Geometry: final body of the model. Coordinates: model frame, mm. Face numbers are marked on the shaded views. A direction names the side the tool comes from. Round coordinates to 2 decimals unless told otherwise and drop trailing zeros. Write each loop counter-clockwise with the first axis right and the second up, starting at its lowest first coordinate (ties: lowest second). Pieces come first, ordered by that corner, then holes. Notation, with made-up numbers: (58, -17.5) - (79, -17.5) arc R31 ccw to (79, 15.5) - close; hole circle Ø6 at (17, 78.5). An arc over 180 degrees is marked (long way). Use a Markdown table: item, result. Add a question column.
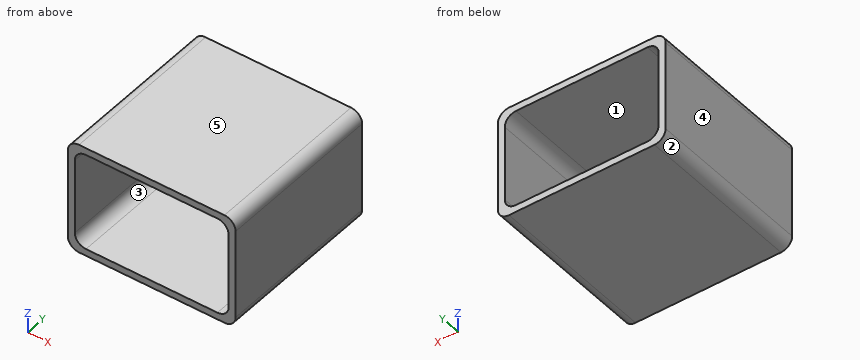
```python
from build123d import *

# Parameters (mm, degrees)
F0_W     = 76.2
F0_H     = 50.8
F1_DEPTH = 76.2
F2_T     = -3.175
F3_R     = 5.08


with BuildPart() as f1:
    # F0 (on Front) → F1 (new body)
    with BuildSketch(Plane.XZ):
        with Locations((7.1646266146, -4.8404615372)):
            Rectangle(F0_W, F0_H)
    extrude(amount=F1_DEPTH)

    # F2
    f2_openings = [f1.faces().sort_by_distance(p)[0] for p in [
        (7.164627, -76.2, -4.840462),
        (7.164627, 0, -4.840462),
    ]]
    offset(amount=F2_T, openings=f2_openings)

    # F3
    f3_edges = [f1.edges().sort_by_distance(p)[0] for p in [
        (45.264627, -38.1, 20.559538),
        (-30.935373, -38.1, 20.559538),
        (45.264627, -38.1, -30.240462),
        (-30.935373, -38.1, -30.240462),
        (42.089627, -38.1, -27.065462),
        (-27.760373, -38.1, -27.065462),
        (-27.760373, -38.1, 17.384538),
        (42.089627, -38.1, 17.384538),
    ]]
    fillet(f3_edges, radius=F3_R)


solid = f1.part
```
1) Set-up query: the marked faces 1 and 2. Return all of +Z, -Z, +X, -X, +Y, -Y with unobstructed straight access to the full face (end or side cutting, diameter ignored); none if empty.
2) Section A-A, the plane x = 13.5. Return the cut outline in (y, z).
3) Section C-C, the plane y = -10.5. Return the cut outline in (x, z), then the cut area to 3 significant figures.
4) Section B-B, the plane z = -6. Return the cut outline in (x, y), then the cut area to 3 significant figures.
5) Material intervals for L1, parallel to Z at x = -21.5, y = -17; L2, parallel to X at y = -49.5, z = -3.5; L3, parallel to Z at x = -23.5, y = -16.5, sorted ascending. Write a range as from..to.
6) Draft query along X for the marked faces 3, 4 and 5. Return one class per face: released by +X, released by -X, zero draft, split by the parting line, or undercut.
Output values:
| question | item | result |
|---|---|---|
| 1 | face 1 | +Y, -Y |
| 1 | face 2 | -Z, -X, +Y, -Y |
| 2 | outline | (-76.2, -30.24) - (0, -30.24) - (0, -27.07) - (-76.2, -27.07) - close; (-76.2, 17.38) - (0, 17.38) - (0, 20.56) - (-76.2, 20.56) - close |
| 3 | outline | (-30.94, -25.16) arc R5.08 ccw to (-25.86, -30.24) - (40.18, -30.24) arc R5.08 ccw to (45.26, -25.16) - (45.26, 15.48) arc R5.08 ccw to (40.18, 20.56) - (-25.86, 20.56) arc R5.08 ccw to (-30.94, 15.48) - close; hole (-27.76, -21.99) arc R5.08 ccw to (-22.68, -27.07) - (37.01, -27.07) arc R5.08 ccw to (42.09, -21.99) - (42.09, 12.3) arc R5.08 ccw to (37.01, 17.38) - (-22.68, 17.38) arc R5.08 ccw to (-27.76, 12.3) - close |
| 3 | area | 766 mm^2 |
| 4 | outline | (-30.94, -76.2) - (-27.76, -76.2) - (-27.76, 0) - (-30.94, 0) - close; (42.09, -76.2) - (45.26, -76.2) - (45.26, 0) - (42.09, 0) - close |
| 4 | area | 484 mm^2 |
| 5 | L1 | z = -30.24..-27.07, 17.38..20.56 |
| 5 | L2 | x = -30.94..-27.76, 42.09..45.26 |
| 5 | L3 | z = -30.24..-27, 17.32..20.56 |
| 6 | face 3 | undercut |
| 6 | face 4 | released by -X |
| 6 | face 5 | zero draft |
